The model under review builds one solid part; all positions refer to its coordinate system, in mm. A direction names the side the tool comes from. Round coordinates to 2 decimals unless told otherwise and drop trailing zeros. Order: outer loops, then holes, each group sorted by start corner. A loop starts at its lowest first (then second) coordinate and runs counter-clockwise, first axis right, second up.
1) Machinability: for faces 4 (the face through (-7, 0, 34)), 5 (the face through (0, -6, 46)), 6 (the face through (-11.25, 0, 15)), 7 (the face through (-10.25, 0, 16)), which of the approach directions +Z, -Z, +X, -X, +Y, -Y give a long, thin tool a straight path to every point of the face, cutting with its end or side? Answer none if there is none.
2) To check wall thickness, follow L1, parallel to X at y = -1.5, z = 52; L2, parallel to X at y = 2, z = 26; L3, parallel to Y at x = -0.5, z = 10.5. State the ranges of each line that lie inside material, in increasing order.
3) Clearance check with flat-ended pins moving along their axes: P1, Ø3, axis at x = -2.5, z = 50.5, coming from the +Y side; P2, Ø3, axis at y = -0.5, z = 51.5, coming from the -X side; P3, Ø5, axis at x = 5.5, z = 44.5, coming from the -Y side; P4, Ø5, axis at x = 6.5, y = 4, coming from the -Z side. State where each tip first meets the part, or that it passes through.
4) Consider section C-C (x = -0.25). Give the boundary of the cut face in (y, z), then the cut area to 3 significant figures.
5) Consider section A-A (z = 50.5). Give the boundary of the cut face in (x, y), then the cut area to 3 significant figures.
6) Consider section B-B (y = 0.25). Give the boundary of the cut face in (x, z), then the cut area to 3 significant figures.
7) Mouldability with a two-part tool opening along Y and no side actions: class faces 1 (the face through (-10.35, 0.1, 33.14)), 2 (the face through (0, -5, 46)), 3 (the face through (-0.157, -6.438, 32.748)) as pulls with the +Y half, pulls with the -Y half, needs draft (parallel to the pull), parting line crosses it, or undercut.
8) Consider section D-D (z = 24.5). Give the boundary of the cut face in (x, y), then the cut area to 3 significant figures.
from build123d import *

# Parameters (mm, degrees)
F0_W         = 12.5
F0_H         = 12
F0_W_2       = 10.5
F0_H_2       = 10
F1_DEPTH     = 62
F0_W_3       = 22.5
F0_H_3       = 14
F0_W_4       = 4
F2_DEPTH     = 34
F3_DEPTH     = 60
F4_DEPTH     = 32
F5_R         = 3
F6_T1_DEPTH  = 29
F6_T6_DEPTH  = 37.5
F6_T11_DEPTH = 37.5
F6_T16_DEPTH = 37.5
F6_T21_DEPTH = 37.5
F6_T26_DEPTH = 37.5
F6_T31_DEPTH = 37.5


# Not quite as in the source:
# - a fillet or chamfer that OpenCascade refuses, or shapes differently, is made with other operations: its cross-section is extruded or revolved along the edge and cut away or added


with BuildPart() as f1:
    # F0 (on Top) → F1 (new body)
    with BuildSketch(Plane.XY):
        Rectangle(F0_W, F0_H)
        Rectangle(F0_W_2, F0_H_2, mode=Mode.SUBTRACT)
        Rectangle(F0_W_2, F0_H_2)
    extrude(amount=F1_DEPTH)

    # F0 (on Top) → F2 (join)
    with BuildSketch(Plane.XY):
        Rectangle(F0_W_3, F0_H_3)
        Polygon((-10.25, -6), (-10.25, 6), (-6.25, 6), (6.25, 6), (10.25, 6), (10.25, -6), (6.25, -6), (-6.25, -6), align=None, mode=Mode.SUBTRACT)
        with Locations((-8.25, 0)):
            Rectangle(F0_W_4, F0_H)
        with Locations((8.25, 0)):
            Rectangle(F0_W_4, F0_H)
    extrude(amount=F2_DEPTH)

    # F0 (on Top) → F3 (cut)
    with BuildSketch(Plane.XY):
        Rectangle(F0_W_2, F0_H_2)
    extrude(amount=F3_DEPTH, mode=Mode.SUBTRACT)

    # F0 (on Top) → F4 (cut)
    with BuildSketch(Plane.XY):
        Rectangle(F0_W, F0_H)
        Rectangle(F0_W_2, F0_H_2, mode=Mode.SUBTRACT)
        with Locations((-8.25, 0)):
            Rectangle(F0_W_4, F0_H)
        with Locations((8.25, 0)):
            Rectangle(F0_W_4, F0_H)
    extrude(amount=F4_DEPTH, mode=Mode.SUBTRACT)

    # F5
    f5_edges = [f1.edges().sort_by_distance(p)[0] for p in [
        (0, 6, 62),
        (-6.25, 0, 62),
        (0, -6, 62),
        (6.25, 0, 62),
    ]]
    fillet(f5_edges, radius=F5_R)

    # F6: fillet of radius 3 on 4 edges, made by hand

    # F6_s2 → F6_t1 (cut)
    with BuildSketch(Plane.XZ.offset(-14.5)):
        with BuildLine():
            ThreePointArc((-8.25, 34), (-10.3713203436, 33.1213203436), (-11.25, 31))
            Line((-11.25, 31), (-11.25, 34))
            Line((-11.25, 34), (-8.25, 34))
        make_face()
        with BuildLine():
            ThreePointArc((8.25, 34), (10.3713203436, 33.1213203436), (11.25, 31))
            Line((11.25, 31), (11.25, 34))
            Line((11.25, 34), (8.25, 34))
        make_face()
    extrude(amount=F6_T1_DEPTH, mode=Mode.SUBTRACT)


with BuildPart() as f6_tool4:
    # F6_s5 → F6_t6 (new body)
    with BuildSketch(Plane.YZ.offset(-18.75)):
        with BuildLine():
            ThreePointArc((-4, 34), (-6.1213203436, 33.1213203436), (-7, 31))
            Line((-7, 31), (-7, 34))
            Line((-7, 34), (-4, 34))
        make_face()
    extrude(amount=F6_T6_DEPTH)

    split(bisect_by=Plane.YZ.offset(-6.25), keep=Keep.BOTTOM)


with BuildPart() as f1_1:
    add(f1.part)

    # F6_t3: cut F6_tool4
    add(f6_tool4.part, mode=Mode.SUBTRACT)


with BuildPart() as f6_tool9:
    # F6_s10 → F6_t11 (new body)
    with BuildSketch(Plane.YZ.offset(-18.75)):
        with BuildLine():
            ThreePointArc((-4, 34), (-6.1213203436, 33.1213203436), (-7, 31))
            Line((-7, 31), (-7, 34))
            Line((-7, 34), (-4, 34))
        make_face()
    extrude(amount=F6_T11_DEPTH)

    split(bisect_by=Plane.XZ.offset(6), keep=Keep.TOP)


with BuildPart() as f1_2:
    add(f1_1.part)

    # F6_t8: cut F6_tool9
    add(f6_tool9.part, mode=Mode.SUBTRACT)


with BuildPart() as f6_tool14:
    # F6_s15 → F6_t16 (new body)
    with BuildSketch(Plane.YZ.offset(-18.75)):
        with BuildLine():
            ThreePointArc((-4, 34), (-6.1213203436, 33.1213203436), (-7, 31))
            Line((-7, 31), (-7, 34))
            Line((-7, 34), (-4, 34))
        make_face()
    extrude(amount=F6_T16_DEPTH)

    split(bisect_by=Plane.YZ.offset(6.25), keep=Keep.TOP)


with BuildPart() as f1_3:
    add(f1_2.part)

    # F6_t13: cut F6_tool14
    add(f6_tool14.part, mode=Mode.SUBTRACT)


with BuildPart() as f6_tool19:
    # F6_s20 → F6_t21 (new body)
    with BuildSketch(Plane.YZ.offset(18.75)):
        with BuildLine():
            ThreePointArc((4, 34), (6.1213203436, 33.1213203436), (7, 31))
            Line((7, 31), (7, 34))
            Line((7, 34), (4, 34))
        make_face()
    extrude(amount=-F6_T21_DEPTH)

    split(bisect_by=Plane.YZ.offset(6.25), keep=Keep.TOP)


with BuildPart() as f1_4:
    add(f1_3.part)

    # F6_t18: cut F6_tool19
    add(f6_tool19.part, mode=Mode.SUBTRACT)


with BuildPart() as f6_tool24:
    # F6_s25 → F6_t26 (new body)
    with BuildSketch(Plane.YZ.offset(18.75)):
        with BuildLine():
            ThreePointArc((4, 34), (6.1213203436, 33.1213203436), (7, 31))
            Line((7, 31), (7, 34))
            Line((7, 34), (4, 34))
        make_face()
    extrude(amount=-F6_T26_DEPTH)

    split(bisect_by=Plane.XZ.offset(-6), keep=Keep.BOTTOM)


with BuildPart() as f1_5:
    add(f1_4.part)

    # F6_t23: cut F6_tool24
    add(f6_tool24.part, mode=Mode.SUBTRACT)


with BuildPart() as f6_tool29:
    # F6_s30 → F6_t31 (new body)
    with BuildSketch(Plane.YZ.offset(18.75)):
        with BuildLine():
            ThreePointArc((4, 34), (6.1213203436, 33.1213203436), (7, 31))
            Line((7, 31), (7, 34))
            Line((7, 34), (4, 34))
        make_face()
    extrude(amount=-F6_T31_DEPTH)

    split(bisect_by=Plane.YZ.offset(-6.25), keep=Keep.BOTTOM)


with BuildPart() as f1_6:
    add(f1_5.part)

    # F6_t28: cut F6_tool29
    add(f6_tool29.part, mode=Mode.SUBTRACT)


solid = f1_6.part
Answer below:
1. face 4: +Z, -X, +Y, -Y
1. face 5: +Z, +X, -X, -Y
1. face 6: +Z, -Z, -X, +Y, -Y
1. face 7: -Z
2. L1: x = -6.25 to -5.25, 5.25 to 6.25
2. L2: x = -11.25 to -10.25, 10.25 to 11.25
2. L3: y = -7 to -6, 6 to 7
3. P1: stops at y = 6
3. P2: stops at x = -6.25
3. P3: stops at y = -6
3. P4: stops at z = 0
4. outline: (-7, 0) - (-6, 0) - (-6, 32) - (-5, 32) - (-5, 60) - (5, 60) - (5, 32) - (6, 32) - (6, 0) - (7, 0) - (7, 31) arc R3 ccw to (6, 33.24) - (6, 59) arc R3 ccw to (3, 62) - (-3, 62) arc R3 ccw to (-6, 59) - (-6, 33.24) arc R3 ccw to (-7, 31) - close
4. area: 141 mm2
5. outline: (-6.25, -6) - (6.25, -6) - (6.25, 6) - (-6.25, 6) - close; hole (-5.25, -5) - (5.25, -5) - (5.25, 5) - (-5.25, 5) - close
5. area: 45.0 mm2
6. outline: (-11.25, 0) - (-10.25, 0) - (-10.25, 32) - (-5.25, 32) - (-5.25, 60) - (5.25, 60) - (5.25, 32) - (10.25, 32) - (10.25, 0) - (11.25, 0) - (11.25, 31) arc R3 ccw to (8.25, 34) - (6.25, 34) - (6.25, 59) arc R3 ccw to (3.25, 62) - (-3.25, 62) arc R3 ccw to (-6.25, 59) - (-6.25, 34) - (-8.25, 34) arc R3 ccw to (-11.25, 31) - close
6. area: 157 mm2
7. face 1: needs draft
7. face 2: undercut
7. face 3: pulls with the -Y half
8. outline: (-11.25, -7) - (11.25, -7) - (11.25, 7) - (-11.25, 7) - close; hole (-10.25, -6) - (10.25, -6) - (10.25, 6) - (-10.25, 6) - close
8. area: 69.0 mm2
